Input: part model. Units: mm. Frame: model coordinates. Face numbers are marked on the shaded views. A direction names the side the tool comes from. Give positions to 0.01 mm unless a question says otherwise; leave off trailing zeros. Loops run counter-clockwise (first coordinate to the right, second up) from the corner with the lowest first, then second, coordinate; pieces in that order, holes last. Notation, with made-up numbers: (-15, 52) - (26, 52) arc R18 cw to (26, 80) - close; hole circle Ø9 at (29, 29.5). An arc over 180 degrees is marked (long way). Answer as a JSON object with one key per item and string values.
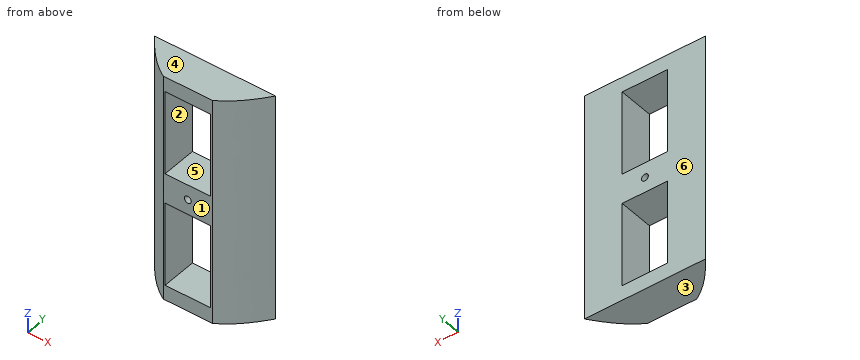
from build123d import *

# Parameters (mm, degrees)
BOSS_EXTRUDE2_DEPTH = 331.382
SKETCH3_R           = 5
SKETCH3_W           = 66
SKETCH3_H           = 122
CUT_EXTRUDE2_DEPTH  = 377.924435453
SKETCH4_W           = 80
SKETCH4_H           = 10
CUT_EXTRUDE3_DEPTH  = 377.924435453
SKETCH5_W           = 260
SKETCH5_H           = 70
CUT_EXTRUDE4_DEPTH  = 377.924435453


with BuildPart() as part:
    # Sketch2 → Boss-Extrude2 (new body)
    with BuildSketch(Plane.XY):
        with BuildLine():
            Line((-127, 127), (127, 127))
            add(Edge.make_bspline(
                [(-127, 127), (0, -127), (127, 127)],
                knots=[0.056028396, 0.056028396, 0.056028396, 0.943971604, 0.943971604, 0.943971604], degree=2))
        make_face()
    extrude(amount=BOSS_EXTRUDE2_DEPTH)

    # Sketch3 → Cut-Extrude2 (cut, through all)
    with BuildSketch(Plane(origin=(0, 127, 0), x_dir=(1, 0, 0), z_dir=(0, 1, 0))):
        with Locations(Location((0, -165.691, 0), (0, 0, 270))):
            Circle(SKETCH3_R)
        with Locations((0, -82.8455)):
            Rectangle(SKETCH3_W, SKETCH3_H)
        with Locations((0, -248.5365)):
            Rectangle(SKETCH3_W, SKETCH3_H)
    extrude(amount=-CUT_EXTRUDE2_DEPTH, mode=Mode.SUBTRACT)

    # Sketch4 → Cut-Extrude3 (cut, through all)
    with BuildSketch(Plane(origin=(0, 0, 0), x_dir=(-1, 0, 0), z_dir=(0, 0, -1))):
        with Locations((0, 5)):
            Rectangle(SKETCH4_W, SKETCH4_H)
    extrude(amount=-CUT_EXTRUDE3_DEPTH, mode=Mode.SUBTRACT)

    # Sketch5 → Cut-Extrude4 (cut, through all)
    with BuildSketch(Plane.XY.offset(331.382)):
        with Locations((0, 95.8)):
            Rectangle(SKETCH5_W, SKETCH5_H)
    extrude(amount=-CUT_EXTRUDE4_DEPTH, mode=Mode.SUBTRACT)


solid = part.part
Item 1: Material intervals for line 1 (Z direction, x = -5.5, y = 31.5); line 2 (X direction, y = 28.5, z = 260); line 3 (X direction, y = 40, z = 25), sorted ascending. Write a range as [from, to].
Geometry check:
{"line 1": "z = [0, 21.85], [143.85, 187.54], [309.54, 331.38]", "line 2": "x = [-60.16, -33], [33, 60.16]", "line 3": "x = [-71.27, -33], [33, 71.27]"}
Item 2: Cut plane A-A (x = 0). Return loops of the section in (y, z).
Geometry check:
{"outline": "(10, 0) - (60.8, 0) - (60.8, 21.85) - (10, 21.85) - close; (10, 143.85) - (60.8, 143.85) - (60.8, 160.69) - (10, 160.69) - close; (10, 170.69) - (60.8, 170.69) - (60.8, 187.54) - (10, 187.54) - close; (10, 309.54) - (60.8, 309.54) - (60.8, 331.38) - (10, 331.38) - close"}
Item 3: Cut plane B-B (x = -22). Return loops of the section in (y, z).
Geometry check:
{"outline": "(10, 0) - (60.8, 0) - (60.8, 21.85) - (10, 21.85) - close; (10, 143.85) - (60.8, 143.85) - (60.8, 187.54) - (10, 187.54) - close; (10, 309.54) - (60.8, 309.54) - (60.8, 331.38) - (10, 331.38) - close"}
Item 4: Cut plane C-C (y = 46). Give the number of separate pieces and of enclosed holes in the cut face, then the cut area to 3 significant figures.
Geometry check:
{"separate pieces": "1", "enclosed holes": "3", "area": "34,500 mm2"}
Item 5: Access query for the marked faces 5 and 6. Directions: +Z, -Z, +X, -X, +Y, -Y. A direction counts if a zero-diameter tool reaches every point of the face in a straight line with its end or side. Return the directions, or none.
Geometry check:
{"face 5": "+Y, -Y", "face 6": "+Z, -Z, +X, -X, +Y"}
Item 6: Contact query for flat-ended pins moving along their axis: P1, Ø15, axis at y = 29, z = 100.5, coming from the -X side; P2, Ø4, axis at y = 25.5, z = 101.5, coming from the +X side; P3, Ø15, axis at y = 27, z = 248, coming from the -X side. Output: stop coordinate, or through.
Geometry check:
{"P1": "stops at x = -68.08", "P2": "stops at x = 59.1", "P3": "stops at x = -66.19"}
Item 7: Mould query, pull axis Z, two halves, no side actions, for the marked faces 1, 2, 3 and 4. Classes: released by +Z, released by -Z, zero draft, split by the parting line, or undercut.
Geometry check:
{"face 1": "zero draft", "face 2": "undercut", "face 3": "released by -Z", "face 4": "released by +Z"}
